from build123d import *

# Parameters (mm, degrees)
F0_W     = 13.9
F0_H     = 13.9
F1_DEPTH = 2
F2_W     = 13.9
F2_H     = 13.9
F3_DEPTH = 5


with BuildPart() as f1:
    # F0 (on Top) → F1 (new body)
    with BuildSketch(Plane.XY):
        Rectangle(F0_W, F0_H)
        with BuildLine():
            ThreePointArc((3.334198, 1.925), (3.718814, 0.996453), (3.85, 0))
            ThreePointArc((3.85, 0), (3.718814, -0.996453), (3.334198, -1.925))
            ThreePointArc((3.334198, -1.925), (1.925, -3.334198), (0, -3.85))
            ThreePointArc((0, -3.85), (-1.925, -3.334198), (-3.334198, -1.925))
            ThreePointArc((-3.334198, -1.925), (-3.85, 0), (-3.334198, 1.925))
            ThreePointArc((-3.334198, 1.925), (-1.925, 3.334198), (0, 3.85))
            ThreePointArc((0, 3.85), (1.925, 3.334198), (3.334198, 1.925))
        make_face(mode=Mode.SUBTRACT)
        with BuildLine():
            ThreePointArc((-3.334198, -1.925), (-1.925, -3.334198), (0, -3.85))
            Line((0, -3.85), (-3.334198, -1.925))
        make_face()
        with BuildLine():
            Line((-3.334198, -1.925), (-3.334198, 1.925))
            ThreePointArc((-3.334198, 1.925), (-3.85, 0), (-3.334198, -1.925))
        make_face()
        with BuildLine():
            Line((-3.334198, 1.925), (0, 3.85))
            ThreePointArc((0, 3.85), (-1.925, 3.334198), (-3.334198, 1.925))
        make_face()
        with BuildLine():
            Line((0, 3.85), (3.334198, 1.925))
            ThreePointArc((3.334198, 1.925), (1.925, 3.334198), (0, 3.85))
        make_face()
        with BuildLine():
            ThreePointArc((3.334198, -1.925), (3.718814, -0.996453), (3.85, 0))
            ThreePointArc((3.85, 0), (3.718814, 0.996453), (3.334198, 1.925))
            Line((3.334198, 1.925), (3.334198, -1.925))
        make_face()
        with BuildLine():
            ThreePointArc((0, -3.85), (1.925, -3.334198), (3.334198, -1.925))
            Line((3.334198, -1.925), (0, -3.85))
        make_face()
    extrude(amount=F1_DEPTH)

    # F2 (on face) → F3 (join)
    with BuildSketch(Plane.XY.offset(2)):
        Rectangle(F2_W, F2_H)
        with BuildLine():
            ThreePointArc((4.330127, 2.5), (4.829629, 1.294095), (5, 0))
            ThreePointArc((5, 0), (4.829629, -1.294095), (4.330127, -2.5))
            ThreePointArc((4.330127, -2.5), (2.5, -4.330127), (0, -5))
            ThreePointArc((0, -5), (-2.5, -4.330127), (-4.330127, -2.5))
            ThreePointArc((-4.330127, -2.5), (-5, 0), (-4.330127, 2.5))
            ThreePointArc((-4.330127, 2.5), (-2.5, 4.330127), (0, 5))
            ThreePointArc((0, 5), (2.5, 4.330127), (4.330127, 2.5))
        make_face(mode=Mode.SUBTRACT)
        with BuildLine():
            Line((-4.330127, -2.5), (-4.330127, 2.5))
            ThreePointArc((-4.330127, 2.5), (-5, 0), (-4.330127, -2.5))
        make_face()
        with BuildLine():
            Line((-4.330127, 2.5), (0, 5))
            ThreePointArc((0, 5), (-2.5, 4.330127), (-4.330127, 2.5))
        make_face()
        with BuildLine():
            Line((0, 5), (4.330127, 2.5))
            ThreePointArc((4.330127, 2.5), (2.5, 4.330127), (0, 5))
        make_face()
        with BuildLine():
            ThreePointArc((4.330127, -2.5), (4.829629, -1.294095), (5, 0))
            ThreePointArc((5, 0), (4.829629, 1.294095), (4.330127, 2.5))
            Line((4.330127, 2.5), (4.330127, -2.5))
        make_face()
        with BuildLine():
            ThreePointArc((0, -5), (2.5, -4.330127), (4.330127, -2.5))
            Line((4.330127, -2.5), (0, -5))
        make_face()
        with BuildLine():
            ThreePointArc((-4.330127, -2.5), (-2.5, -4.330127), (0, -5))
            Line((0, -5), (-4.330127, -2.5))
        make_face()
    extrude(amount=F3_DEPTH)


solid = f1.part
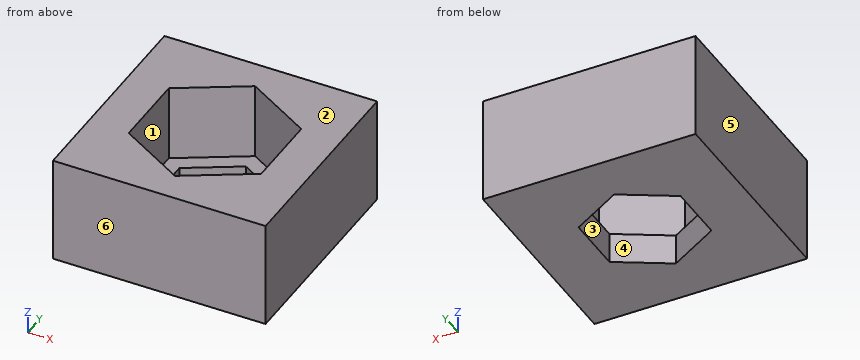
CAD build for the part. Positions are in the model's coordinates, mm. Face numbers are marked on the shaded views. A direction names the side the tool comes from. Round coordinates to 2 decimals unless told otherwise and drop trailing zeros. Write each loop counter-clockwise with the first axis right and the second up, starting at its lowest first coordinate (ties: lowest second). Pieces come first, ordered by that corner, then holes.
(1) Drop a flat-ended pin along its axis: P1, Ø3, axis at x = -0.5, y = -3.5, coming from the -Z side. Give the stop position or say it passes through.
(2) Probe line 1 along X through (y, z) = (-1.75, 1); line 2 along Y through (x, z) = (-2, 4); line 3 along X through (y, z) = (-0.5, 6.5). List the from-to ranges inside material, lowest first.
(3) 3-axis set-ups, long thin cutter, end or side, ignore diameter. For the marked faces 1, 2 and 3: which of +Z, -Z, +X, -X, +Y, -Y reach the whole face in a straight line?
(4) Slice it at D-D, the plane z = 5.75. Write the cut outline in (x, y), and give its area (3 significant figures).
(5) Slice it at C-C, the plane x = -2.5. Write the cut outline in (y, z).
(6) Slice it at A-A, the plane y = -0.75. Write the cut outline in (x, z), and give its area (3 significant figures).
(7) Mould opens along X. For the marked faces 4, 5 and 6 say: pulls with the +X half, pulls with the -X half, needs draft (parallel to the pull), parting line crosses it, or undercut.
(8) Slice it at B-B, the plane z = 1.5. Write the cut outline in (x, y) (3 decimals), and give its area (3 significant figures).
From the geometry:
1. P1: stops at z = 0
2. line 1: x = -6.95 to -3.33, 3.33 to 6.95
2. line 2: y = -6.95 to -3.85, 3.85 to 6.95
2. line 3: x = -6.95 to -4.33, 4.33 to 6.95
3. face 1: +Z
3. face 2: +Z, +X, -X, +Y, -Y
3. face 3: +Z, -Z
4. outline: (-6.95, -6.95) - (6.95, -6.95) - (6.95, 6.95) - (-6.95, 6.95) - close; hole (-4.33, -2.5) - (0, -5) - (4.33, -2.5) - (4.33, 2.5) - (0, 5) - (-4.33, 2.5) - close
4. area: 128 mm2
5. outline: (-6.95, 0) - (-2.41, 0) - (-2.41, 2) - (-3.56, 2) - (-3.56, 7) - (-6.95, 7) - close; (2.41, 0) - (6.95, 0) - (6.95, 7) - (3.56, 7) - (3.56, 2) - (2.41, 2) - close
6. outline: (-6.95, 0) - (-3.33, 0) - (-3.33, 2) - (-4.33, 2) - (-4.33, 7) - (-6.95, 7) - close; (3.33, 0) - (6.95, 0) - (6.95, 7) - (4.33, 7) - (4.33, 2) - (3.33, 2) - close
6. area: 40.7 mm2
7. face 4: undercut
7. face 5: pulls with the -X half
7. face 6: needs draft
8. outline: (-6.95, -6.95) - (6.95, -6.95) - (6.95, 6.95) - (-6.95, 6.95) - close; hole (-3.334, -1.925) - (0, -3.85) - (3.334, -1.925) - (3.334, 1.925) - (0, 3.85) - (-3.334, 1.925) - close
8. area: 155 mm2
